```python
from build123d import *

# Parameters (mm, degrees)
F1_DEPTH = 25.4
F2_R     = 25.4
F3_R     = 12.7
F4_DEPTH = 25.4


with BuildPart() as f1:
    # F0 (on Right) → F1 (new body)
    with BuildSketch(Plane.YZ):
        Polygon((50.8, -76.2), (50.8, 76.2), (50.8, 87.988181), (-101.6, 0), (50.8, -87.988181), align=None)
    extrude(amount=F1_DEPTH)

    # F2
    f2_edges = [f1.edges().sort_by_distance(p)[0] for p in [
        (12.7, -101.6, 0),
    ]]
    fillet(f2_edges, radius=F2_R)

    # F3 (on face) → F4 (cut)
    with BuildSketch(Plane.YZ.offset(25.4)):
        with Locations((-50.8, 0)):
            Circle(F3_R)
    extrude(amount=-F4_DEPTH, mode=Mode.SUBTRACT)


solid = f1.part
```
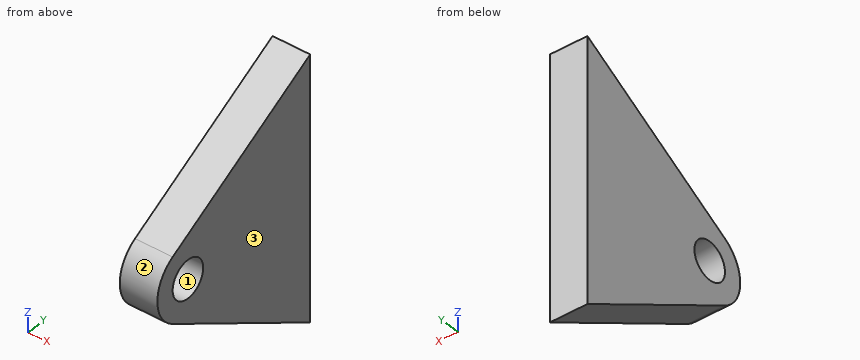
Geometry check sheet. Reference: the model listing, model coordinates, mm. Face numbers are marked on the shaded views. Give positions to 0.01 mm unless a question says otherwise; leave off trailing zeros. Order: outer loops, then holes, each group sorted by start corner. A loop starts at its lowest first (then second) coordinate and runs counter-clockwise, first axis right, second up. Notation, with made-up numbers: (55.5, -7) - (110.5, -7) arc R16 ccw to (110.5, 20) - close; hole circle Ø9 at (50.25, 14). An arc over 180 degrees is marked (long way). Answer in a Markdown table with one row per item. Add a question column.
Q1. Gauge pin test, flat ends, axial feed: pin 1 (1 mm diameter, centred on x = 5, y = 30, fed in from +Z); pin 2 (1 mm diameter, centred on x = 13.5, z = 42, fed in from -Y); pin 3 (1 mm diameter, centred on x = 5.5, y = 1, fed in from +Z). Record the tip position at first contact, or that the pin passes through.
Q2. Mould release check, pull along Y, two halves, no side actions. Record for the marked faces 1, 2 and 3: pulls with the +Y half, pulls with the -Y half, needs draft (parallel to the pull), parting line crosses it, or undercut.
Q3. Cross-section at D-D, the plane y = 23.5. Enter the section's corners in (x, z).
Q4. Cross-section at B-B, the plane x = 21.5. Enter the section's corners in (y, z), then the cut area to 3 significant figures.
Q5. Material ranges on probe 1 along Z at (x, y) = (10.5, -59); probe 2 along Z at (x, y) = (11.25, -50.8); probe 3 along Y at (x, z) = (1.75, 9), recorded low to high. Write a range as from..to.
Q6. Cross-section at A-A, the plane z = 0. Enter the section's corners in (x, y), then the cut area to 3 significant figures.
Q7. Cross-section at C-C, the plane y = -50.8. Enter the section's corners in (x, z).
Check values:
| question | item | result |
|---|---|---|
| 1 | pin 1 | stops at z = 76.27 |
| 1 | pin 2 | stops at y = -29.72 |
| 1 | pin 3 | stops at z = 59.52 |
| 2 | face 1 | undercut |
| 2 | face 2 | pulls with the -Y half |
| 2 | face 3 | needs draft |
| 3 | outline | (0, -72.23) - (25.4, -72.23) - (25.4, 72.23) - (0, 72.23) - close |
| 4 | outline | (-63.5, -22) - (50.8, -87.99) - (50.8, 87.99) - (-63.5, 22) arc R25.4 ccw to start; hole circle Ø25.4 at (-50.8, 0) |
| 4 | area | 12,500 mm^2 |
| 5 | probe 1 | z = -24.6..-9.7, 9.7..24.6 |
| 5 | probe 2 | z = -29.33..-12.7, 12.7..29.33 |
| 5 | probe 3 | y = -74.55..-59.76, -41.84..50.8 |
| 6 | outline | (0, -76.2) - (25.4, -76.2) - (25.4, -63.5) - (0, -63.5) - close; (0, -38.1) - (25.4, -38.1) - (25.4, 50.8) - (0, 50.8) - close |
| 6 | area | 2,580 mm^2 |
| 7 | outline | (0, -29.33) - (25.4, -29.33) - (25.4, -12.7) - (0, -12.7) - close; (0, 12.7) - (25.4, 12.7) - (25.4, 29.33) - (0, 29.33) - close |
